Build history of the part. All positions in model axes, mm. A direction names the side the tool comes from. Round coordinates to 2 decimals unless told otherwise and drop trailing zeros. Write each loop counter-clockwise with the first axis right and the second up, starting at its lowest first coordinate (ties: lowest second). Pieces come first, ordered by that corner, then holes. Notation, with made-up numbers: M 30,31.25 L 46,31.25 A33 cw 46,62.25 Z; hole C -26.5,76 d2. An arc over 180 degrees is marked long. Write item = value, one per line. Start each with the question number.
Q1. Tool access for faces 1 (the flat face through (-1.07, -2.969, -1.756)), 2 (the flat face through (-1.07, 2.969, 1.756)), 3 (the flat face through (-1.1, 3, -1.7)), 4 (the flat face through (-1.1, -3, 1.7)): list every direction of +Z, -Z, +X, -X, +Y, -Y with a clear straight run to the whole face (end or side of a thin tool).
Q2. Pull direction Y, two halves, no side cores. Call faces 5 (the cylindrical face through (5.014, 7.167, -4.57)), 6 (the flat face through (4, 0, -4)), 7 (the cylindrical face through (-0.084, -0.67, 1.617)): released by +Y, released by -Y, zero draft, split by the parting line, or undercut.
Q3. Probe L1, parallel to Y at x = -2.75, z = 0; L2, parallel to Z at x = -3.25, y = 1; L3, parallel to X at y = 5.75, z = -1.5. List the from-to ranges inside material, lowest first.
Q4. Band-saw the part on D-D on z = 2.5. Write the cut outline in (x, y), plus the area to 3 significant figures.
Q5. Band-saw the part on C-C on z = 0.25. Write the cut outline in (x, y).
Q6. Drop flat-ended pins along their axis: P1, Ø2, axis at x = 2, z = -6.5, coming from the -Y side; P2, Ø5, axis at x = 2.5, y = 1, coming from the -Z side; P3, Ø1, axis at x = -2, y = 2, coming from the -Z side; P4, Ø6, axis at x = -4, z = 6, coming from the -Y side. Give the stop position or say it passes through.
Q7. Band-saw the part on A-A on x = 2. Write the cut outline in (y, z).
Q8. Band-saw the part on B-B on y = 0.75. Write the cut outline in (x, z).
Autodesk Inventor part; units mm, degrees
ref_plane "YZ Plane" through (0, 0, 0) normal (1, 0, 0) x (0, 1, 0)
ref_plane "XZ Plane" through (0, 0, 0) normal (0, 1, 0) x (-1, 0, 0)
ref_plane "XY Plane" through (0, 0, 0) normal (0, 0, 1) x (1, 0, 0)
sketch "Sketch1" plane through (0, 0, 0) normal (1, 0, 0) x (0, 1, 0)
  line L0 (2, 0) -> (-2, 0) construction
  line L1 (-2, 0) -> (-2, -15.7322) construction
  line L2 (-2, -15.7322) -> (2, -15.7322) construction
  line L3 (2, -15.7322) -> (2, 0) construction
  line L4 (2, -3.4446) -> (-1.9831, -3.4544)
  line L5 (-1.9831, -3.4544) -> (-3.9831, -0.0097)
  line L6 (-3.9831, -0.0097) -> (-2, 3.4446)
  line L7 (-2, 3.4446) -> (1.9831, 3.4544)
  line L8 (1.9831, 3.4544) -> (3.9831, 0.0097)
  line L9 (3.9831, 0.0097) -> (2, -3.4446)
  point P0 (0, 0)
  point P1 (0, 0)
  dimension "d0" = 4
extrude "Extrusion1" add sketch "Sketch1" along normal blind 4 and the other way blind 6
sketch "Sketch2" plane through (4, 0, 0) normal (1, 0, 0) x (0, 0, -1)
  line L0 (3.4446, 2) -> (-0.0097, 3.9831)
  circle A0 centre (0, 0) radius 3.9832
extrude "Extrusion2" add sketch "Sketch2" along normal blind 2
sketch "Sketch3" plane through (6, 0, 0) normal (1, 0, 0) x (0, 0, -1)
  point P0 (0, 0)
sketch "Sketch4" plane through (4, 0, 0) normal (-1, 0, 0) x (0, 0, 1)
  circle A0 centre (0, 0) radius 6
  dimension "d5" = 12
extrude "Extrusion3" add sketch "Sketch4" against normal blind 2
sketch "Sketch5" plane through (6, 0, 0) normal (1, 0, 0) x (0, 0, -1)
  circle A0 centre (0, 0) radius 1.5
  dimension "d8" = 3
extrude "Extrusion4" cut sketch "Sketch5" against normal blind 6
sketch "Sketch6" plane through (6, 0, 0) normal (1, 0, 0) x (0, 0, -1)
  point P0 (0, 0)
sketch "Sketch7" plane through (6, 0, 0) normal (1, 0, 0) x (0, 0, -1)
  circle A0 centre (0, 0) radius 8.5
  dimension "d11" = 17
extrude "Extrusion5" add sketch "Sketch7" against normal blind 2
sketch "Sketch8" plane through (-6, 0, 0) normal (-1, 0, 0) x (0, 0, 1)
  circle A0 centre (0, 0) radius 1.75
  dimension "d16" = 3.5
extrude "Extrusion6" cut sketch "Sketch8" against normal blind 12.25
properties part number "InnerLayerHub3mm"
Conclusion:
q1.face_1 = -Z, -X, -Y
q1.face_2 = +Z, -X, +Y
q1.face_3 = -Z, -X, +Y
q1.face_4 = +Z, -X, -Y
q2.face_5 = split by the parting line
q2.face_6 = zero draft
q2.face_7 = undercut
q3.L1 = -3.98 to -1.75, 1.75 to 3.98
q3.L2 = -3.45 to -1.44, 1.44 to 3.45
q3.L3 = 4 to 6
q4.outline = M -6,-2.54 L 4,-2.54 L 4,-8.12 L 6,-8.12 L 6,8.12 L 4,8.12 L 4,2.54 L -6,2.54 Z
q4.area = 83.3 mm^2
q5.outline = M -6,-3.83 L 4,-3.83 L 4,-8.5 L 6,-8.5 L 6,-1.73 L -6,-1.73 Z; M -6,1.73 L 6,1.73 L 6,8.5 L 4,8.5 L 4,3.84 L -6,3.84 Z
q6.P1 = through
q6.P2 = -8.5
q6.P3 = -3.45
q6.P4 = -2.26
q7.outline = M -3.98,-0.01 L -1.98,-3.45 L 2,-3.44 L 3.98,0.01 L 1.98,3.45 L -2,3.44 Z; hole C 0,0 d3.5
q8.outline = M -6,-3.45 L 4,-3.45 L 4,-8.47 L 6,-8.47 L 6,-1.58 L -6,-1.58 Z; M -6,1.58 L 6,1.58 L 6,8.47 L 4,8.47 L 4,3.45 L -6,3.45 Z
